Geometry check sheet. Reference: the model listing, model coordinates, mm. Round coordinates to 2 decimals unless told otherwise and drop trailing zeros. Write each loop counter-clockwise with the first axis right and the second up, starting at its lowest first coordinate (ties: lowest second). Pieces come first, ordered by that corner, then holes.
from build123d import *

# Parameters (mm, degrees)
BASPROSKE_W             = 5
BASPROSKE_H             = 6.5
TOOTHCUT_DEPTH          = 11.464224768
TEETHCUTS_COUNT         = 11
TEETHCUTS_ANGLE         = 327.272727273
BORSKE_R                = 1.5
BORE_DEPTH              = 50.0000508
ESQUISSE1_R             = 2.75
ENL_V_MAT_EXTRU_1_DEPTH = 3
ESQUISSE2_R             = 2.75
ESQUISSE2_R_2           = 1.5
BOSS_EXTRU_1_DEPTH      = 3
ENL_V_MAT_EXTRU_2_DEPTH = 2
BOSS_EXTRU_2_START      = -2
ESQUISSE4_R             = 3.301127001
ESQUISSE4_R_2           = 1.5
BOSS_EXTRU_2_DEPTH      = 2
ENL_V_MAT_EXTRU_3_DEPTH = 2.5


with BuildPart() as part:
    # BasProSke → Base-Revolve (revolve)
    with BuildSketch(Plane(origin=(0, 0, 0), x_dir=(1, 0, 0), z_dir=(0, 1, 0)), mode=Mode.PRIVATE) as base_revolve_sk:
        with Locations((2.5, 3.25)):
            Rectangle(BASPROSKE_W, BASPROSKE_H)
    revolve(base_revolve_sk.sketch.rotate(Axis((-10, 0, 0), (1, 0, 0)), 180), axis=Axis((-10, 0, 0), (1, 0, 0)))

    # TooCutSke → ToothCut (cut, through all)
    with BuildSketch(Plane(origin=(0, 0, 0), x_dir=(0, 0, -1), z_dir=(1, 0, 0))):
        with BuildLine():
            ThreePointArc((0.576045815, 4.209771041), (0, 4.249), (-0.576045815, 4.209771041))
            ThreePointArc((-0.576045815, 4.209771041), (-0.841371334, 5.420048739), (-1.718652745, 6.295004202))
            ThreePointArc((-1.718652745, 6.295004202), (0, 6.5254), (1.718652745, 6.295004202))
            ThreePointArc((1.718652745, 6.295004202), (0.841371334, 5.420048739), (0.576045815, 4.209771041))
        make_face()
    toothcut = extrude(amount=TOOTHCUT_DEPTH, mode=Mode.SUBTRACT)

    # TeethCuts: ToothCut ×11 about axis
    teethcuts_axis = Axis((-10, 0, 0), (1, 0, 0))
    for i in range(1, TEETHCUTS_COUNT):
        add(toothcut.rotate(teethcuts_axis, i * TEETHCUTS_ANGLE / (TEETHCUTS_COUNT - 1)), mode=Mode.SUBTRACT)

    # BorSke → Bore (cut, symmetric)
    with BuildSketch(Plane(origin=(0, 0, 0), x_dir=(0, 0, -1), z_dir=(1, 0, 0))):
        with Locations(Location((0, 0, 0), (0, 0, 180))):
            Circle(BORSKE_R)
    extrude(amount=BORE_DEPTH, both=True, mode=Mode.SUBTRACT)

    # Esquisse1 → Enlèv. mat.-Extru.1 (cut)
    with BuildSketch(Plane.ZY):
        Circle(ESQUISSE1_R)
    extrude(amount=-ENL_V_MAT_EXTRU_1_DEPTH, mode=Mode.SUBTRACT)

    # Esquisse2 → Boss.-Extru.1 (add)
    with BuildSketch(Plane.ZY.offset(-3)):
        Circle(ESQUISSE2_R)
        Circle(ESQUISSE2_R_2, mode=Mode.SUBTRACT)
    extrude(amount=BOSS_EXTRU_1_DEPTH)

    # Esquisse3 → Enlèv. mat.-Extru.2 (cut)
    with BuildSketch(Plane.ZY):
        Polygon((2.381429268, -2.186807713), (3.084545667, 0.968974387), (0.703116398, 3.1557821), (-2.381429268, 2.186807713), (-3.084545667, -0.968974387), (-0.703116398, -3.1557821), align=None)
    extrude(amount=-ENL_V_MAT_EXTRU_2_DEPTH, mode=Mode.SUBTRACT)

    # Esquisse4 → Boss.-Extru.2 (add)
    with BuildSketch(Plane.ZY.offset(BOSS_EXTRU_2_START)):
        Circle(ESQUISSE4_R)
        Circle(ESQUISSE4_R_2, mode=Mode.SUBTRACT)
    extrude(amount=BOSS_EXTRU_2_DEPTH)

    # Esquisse5 → Enlèv. mat.-Extru.3 (cut)
    with BuildSketch(Plane.ZY):
        with BuildLine():
            Line((-1.61510442, 2.41463511), (2.872559283, 0.432929749))
            ThreePointArc((2.872559283, 0.432929749), (-1.173493595, -2.657430673), (-1.61510442, 2.41463511))
        make_face()
    extrude(amount=-ENL_V_MAT_EXTRU_3_DEPTH, mode=Mode.SUBTRACT)


solid = part.part
1. Depth check by flat-ended pin: pin 1 Ø2 at (y, z) = (-4, 3.5) entering from -X; pin 2 Ø3 at (x, y) = (1.5, -2) entering from +Z; pin 3 Ø1 at (x, y) = (4.5, -3) entering from -Z. Enter the tip coordinate at first touch or a pass-through.
2. Section check A-A (y = -0.25). Record the cut outline in (x, z).
3. Section check D-D (y = 2.75). Record the cut outline in (x, z).
4. Section check B-B (y = 5.75). Record the cut outline in (x, z), plus the area to 3 significant figures.
5. Scan lines: line 1 along Z through (x, y) = (1.9, -2.5); line 2 along Z through (x, y) = (0.35, 3.5); line 3 along Y through (x, z) = (1, -4.5). Record each from-to range of solid material in increasing order.
6. Section check C-C (y = -2). Record the cut outline in (x, z).
Results below:
1. pin 1: stops at x = 0
1. pin 2: stops at z = 5.97
1. pin 3: stops at z = -5.97
2. outline: (0, -4.24) - (5, -4.24) - (5, -1.48) - (2.5, -1.48) - (2.5, -2.89) - (0, -2.89) - close; (0, 2.89) - (2.5, 2.89) - (2.5, 1.48) - (5, 1.48) - (5, 4.24) - (0, 4.24) - close
3. outline: (0, -4.35) - (5, -4.35) - (5, 4.35) - (0, 4.35) - close
4. outline: (0, -2.15) - (5, -2.15) - (5, -1.06) - (0, -1.06) - close; (0, 1.06) - (5, 1.06) - (5, 2.15) - (0, 2.15) - close
4. area: 10.9 mm2
5. line 1: z = -5.95 to -3.76, -3.44 to -1.48, 1.48 to 3.44, 3.76 to 5.95
5. line 2: z = -4.85 to -2.94, -2.41 to 2.41, 2.94 to 4.85
5. line 3: y = -2.88 to -1.24, -0.07 to 1.4, 2.92 to 4.36
6. outline: (0, -5.65) - (5, -5.65) - (5, 5.65) - (0, 5.65) - (0, 2.11) - (2.5, 2.11) - (2.5, -2.11) - (0, -2.11) - close
